```python
from build123d import *

# Parameters (mm, degrees)
BOSS_EXTRUDE4_DEPTH = 50
SKETCH7_R           = 1.75
CUT_EXTRUDE1_DEPTH  = 17.825
SKETCH8_R           = 0.75
SKETCH8_W           = 11.8
SKETCH8_H           = 22.5
BOSS_EXTRUDE5_DEPTH = 6
SKETCH9_R           = 7.5
BOSS_EXTRUDE6_DEPTH = 8
FILLET1_R           = 2
SKETCH10_R          = 4.5
CUT_EXTRUDE2_DEPTH  = 65


with BuildPart() as part:
    # Sketch6 → Boss-Extrude4 (new body)
    with BuildSketch(Plane.XZ):
        with BuildLine():
            Line((-1, 25.784833184), (-1, 12.785954208))
            ThreePointArc((-1, 12.785954208), (-12.825, 0), (-1, -12.785954208))
            Line((-1, -12.785954208), (-1, -25.784833184))
            Line((-1, -25.784833184), (-6, -25.784833184))
            Line((-6, -25.784833184), (-6, -16.784833184))
            ThreePointArc((-6, -16.784833184), (-17.825, 0), (-6, 16.784833184))
            Line((-6, 16.784833184), (-6, 25.784833184))
            Line((-6, 25.784833184), (-1, 25.784833184))
        make_face()
    extrude(amount=BOSS_EXTRUDE4_DEPTH)

    # Sketch7 → Cut-Extrude1 (cut, through all)
    with BuildSketch(Plane(origin=(-1, 0, 0), x_dir=(0, 0, -1), z_dir=(1, 0, 0))):
        with Locations((-19.285393696, -10)):
            Circle(SKETCH7_R)
        with Locations((-19.285393696, -40)):
            Circle(SKETCH7_R)
        with Locations((19.285393696, -40)):
            Circle(SKETCH7_R)
        with Locations((19.285393696, -10)):
            Circle(SKETCH7_R)
    extrude(amount=-CUT_EXTRUDE1_DEPTH, mode=Mode.SUBTRACT)

    # Sketch8 → Boss-Extrude5 (add)
    with BuildSketch(Plane(origin=(0, 0, 0), x_dir=(1, 0, 0), z_dir=(0, 1, 0))):
        with BuildLine():
            Line((-35.384131785, -16.25), (-22.318992281, -16.25))
            ThreePointArc((-22.318992281, -16.25), (-21.069616181, -16.522536094), (-20.047240136, -17.290627093))
            ThreePointArc((-20.047240136, -17.290627093), (26.473715688, 0), (-20.047240136, 17.290627093))
            ThreePointArc((-20.047240136, 17.290627093), (-21.069616181, 16.522536094), (-22.318992281, 16.25))
            Line((-22.318992281, 16.25), (-35.384131785, 16.25))
            ThreePointArc((-35.384131785, 16.25), (-37.505452129, 15.371320344), (-38.384131785, 13.25))
            Line((-38.384131785, 13.25), (-38.384131785, -13.25))
            ThreePointArc((-38.384131785, -13.25), (-37.505452129, -15.371320344), (-35.384131785, -16.25))
        make_face()
        with Locations((-27.484131785, 13.65)):
            Circle(SKETCH8_R, mode=Mode.SUBTRACT)
        with Locations((-27.484131785, -13.65)):
            Circle(SKETCH8_R, mode=Mode.SUBTRACT)
        with Locations((-27.484131785, 0)):
            Rectangle(SKETCH8_W, SKETCH8_H, mode=Mode.SUBTRACT)
    extrude(amount=BOSS_EXTRUDE5_DEPTH)

    # Sketch9 → Boss-Extrude6 (add)
    with BuildSketch(Plane(origin=(0, 6, 0), x_dir=(1, 0, 0), z_dir=(0, 1, 0))):
        Circle(SKETCH9_R)
    extrude(amount=BOSS_EXTRUDE6_DEPTH)

    # Fillet1
    fillet1_edges = [part.edges().sort_by_distance(p)[0] for p in [
        (-7.5, 6, 0),
    ]]
    fillet(fillet1_edges, radius=FILLET1_R)

    # Sketch10 → Cut-Extrude2 (cut, through all)
    with BuildSketch(Plane(origin=(0, 14, 0), x_dir=(1, 0, 0), z_dir=(0, 1, 0))):
        Circle(SKETCH10_R)
    extrude(amount=-CUT_EXTRUDE2_DEPTH, mode=Mode.SUBTRACT)


solid = part.part
```
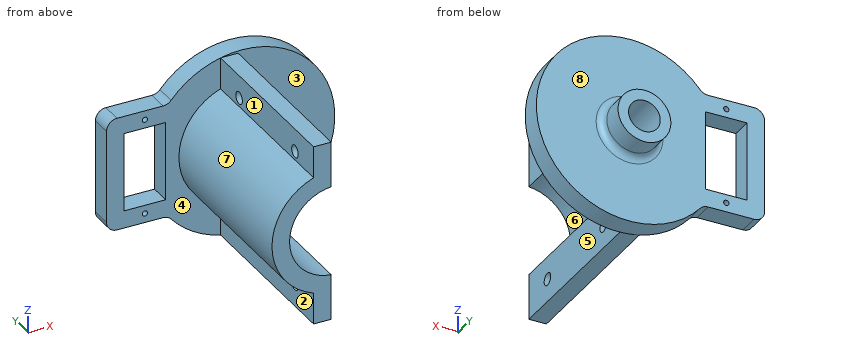
CAD build for the part. Positions are in the model's coordinates, mm. Face numbers are marked on the shaded views. A direction names the side the tool comes from. Give positions to 0.01 mm unless a question says otherwise; leave off trailing zeros. Order: outer loops, then holes, each group sorted by start corner. A loop starts at its lowest first (then second) coordinate and runs counter-clockwise, first axis right, second up.
(1) Drill centre lines: L1, parallel to Z at x = 0, y = 5; L2, parallel to Z at x = -11, y = -16.5; L3, parallel to Y at x = -16, z = 21. Where is each one in solid material? Low to high.
(2) Flat gauge pins, fed straight in: pin 1 (5.5 mm diameter, centred on y = -10, z = -19.29, fed in from -X); pin 2 (1.5 mm diameter, centred on x = -4, z = 18, fed in from +Y); pin 3 (9.5 mm diameter, centred on x = -26, z = -11, fed in from -Y); pin 4 (0.9 mm diameter, centred on x = -27.48, z = -13.65, fed in from +Y). Where does each tip first touch, or does it go through?
(3) Mould opens along Z. For the marked faces 6, 7 and 8 say: released by +Z, released by -Z, zero draft, split by the parting line, or undercut.
(4) Saw through at A-A, the plane z = 0. Give the cut face in (x, y) (3 decimals).
(5) Saw through at D-D, the plane z = 23. Give the cut face in (x, y), then the cut area to 3 significant figures.
(6) Tool access for the marked faces 1, 2, 3, 4 and 5: list every direction of +Z, -Z, +X, -X, +Y, -Y with a clear straight run to the whole face (end or side of a thin tool).
(7) Saw through at B-B, the plane y = -10. Give the cut face in (x, z) (3 decimals).
(8) Saw through at C-C, the plane x = -11. Give the cut face in (y, z), then the cut area to 3 significant figures.
Results found:
1. L1: z = -26.47 to -4.5, 4.5 to 26.47
1. L2: z = -14.03 to -6.59, 6.59 to 14.03
1. L3: y = 0 to 6
2. pin 1: stops at x = -6.65
2. pin 2: stops at y = 6
2. pin 3: stops at y = 0
2. pin 4: passes through
3. face 6: undercut
3. face 7: split by the parting line
3. face 8: zero draft
4. outline: (-38.384, 0) - (-33.384, 0) - (-33.384, 6) - (-38.384, 6) - close; (-21.584, 0) - (-17.825, 0) - (-17.825, -50) - (-12.825, -50) - (-12.825, 0) - (-4.5, 0) - (-4.5, 14) - (-7.5, 14) - (-7.5, 8) arc R2 cw to (-9.5, 6) - (-21.584, 6) - close; (4.5, 0) - (26.474, 0) - (26.474, 6) - (9.5, 6) arc R2 cw to (7.5, 8) - (7.5, 14) - (4.5, 14) - close
5. outline: (-13.11, 0) - (-6, 0) - (-6, -50) - (-1, -50) - (-1, 0) - (13.11, 0) - (13.11, 6) - (-13.11, 6) - close
5. area: 407 mm2
6. face 1: +Z, -X, -Y
6. face 2: -Z, -X, -Y
6. face 3: +X, -Y
6. face 4: -X, -Y
6. face 5: +Z, -Z, +X, -Y
7. outline: (-6, -25.785) - (-1, -25.785) - (-1, -21.035) - (-6, -21.035) - close; (-6, -17.535) - (-1, -17.535) - (-1, -12.786) arc R12.825 cw to (-1, 12.786) - (-1, 17.535) - (-6, 17.535) - (-6, 16.785) arc R17.825 ccw to (-6, -16.785) - close; (-6, 21.035) - (-1, 21.035) - (-1, 25.785) - (-6, 25.785) - close
8. outline: (-50, -14.03) - (0, -14.03) - (0, -24.08) - (6, -24.08) - (6, 24.08) - (0, 24.08) - (0, 14.03) - (-50, 14.03) - (-50, 6.59) - (0, 6.59) - (0, -6.59) - (-50, -6.59) - close
8. area: 1,030 mm2
